CAD build for the part. Positions are in the model's coordinates, mm. Face numbers are marked on the shaded views. A direction names the side the tool comes from. Coordinates: 2 decimals unless noted, no trailing zeros. Loops run counter-clockwise (first coordinate to the right, second up) from the corner with the lowest first, then second, coordinate; pieces in that order, holes last. Notation, with made-up numbers: (-31.5, -5) -> (24.5, -5) arc R16 cw to (24.5, 18) -> close; hole circle Ø8 at (59, 5). An arc over 180 degrees is marked (long way). Write each question's results on one line, items separated by ' | '.
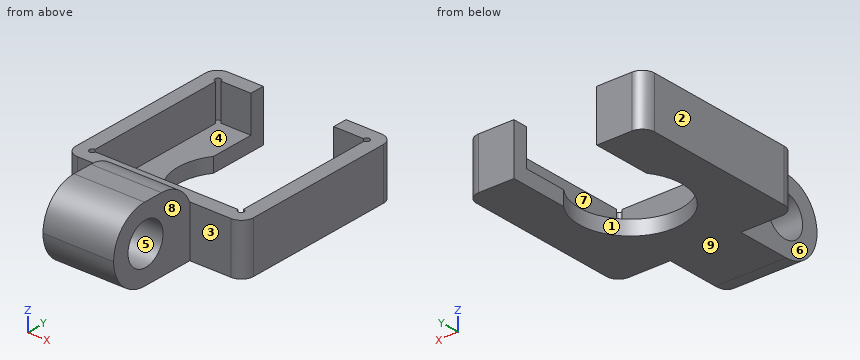
from build123d import *

# Parameters (mm, degrees)
F1_DEPTH    = 1.2
F2_DEPTH    = 4.2
F3_DEPTH    = 6
F6_T1_DEPTH = 20.8
F6_T3_DEPTH = 19.5477270849
F7_D        = 3.4
F7_DEPTH    = 7
F7_TIP      = 1.0214630523
F8_R        = 1


# Not quite as in the source:
# - a fillet or chamfer that OpenCascade refuses, or shapes differently, is made with other operations: its cross-section is extruded or revolved along the edge and cut away or added


with BuildPart() as f1:
    # F0 (on Top) → F1 (new body)
    with BuildSketch(Plane.XY):
        with BuildLine():
            Line((-3.4, 6.1), (-5.85, 6.1))
            ThreePointArc((-5.85, 6.1), (-6.2767766953, 6.2767766953), (-6.1, 5.85))
            Line((-6.1, 5.85), (-6.1, -5.85))
            ThreePointArc((-6.1, -5.85), (-6.2767766953, -6.2767766953), (-5.85, -6.1))
            Line((-5.85, -6.1), (5.85, -6.1))
            ThreePointArc((5.85, -6.1), (6.2767766953, -6.2767766953), (6.1, -5.85))
            Line((6.1, -5.85), (6.1, 5.85))
            ThreePointArc((6.1, 5.85), (6.2767766953, 6.2767766953), (5.85, 6.1))
            Line((5.85, 6.1), (3.4, 6.1))
            Line((3.4, 6.1), (3.4, 2.4657656012))
            ThreePointArc((3.4, 2.4657656012), (0, -4.2), (-3.4, 2.4657656012))
            Line((-3.4, 2.4657656012), (-3.4, 6.1))
        make_face()
    extrude(amount=F1_DEPTH)

    # F0 (on Top) → F2 (join)
    with BuildSketch(Plane.XY):
        with BuildLine():
            ThreePointArc((-6.1, 5.85), (-6.2767766953, 6.2767766953), (-5.85, 6.1))
            Line((-5.85, 6.1), (-3.4, 6.1))
            Line((-3.4, 6.1), (-3.4, 7.3))
            Line((-3.4, 7.3), (-7.3, 7.3))
            Line((-7.3, 7.3), (-7.3, -7.3))
            Line((-7.3, -7.3), (-2.9, -7.3))
            Line((-2.9, -7.3), (2.9, -7.3))
            Line((2.9, -7.3), (7.3, -7.3))
            Line((7.3, -7.3), (7.3, 7.3))
            Line((7.3, 7.3), (3.4, 7.3))
            Line((3.4, 7.3), (3.4, 6.1))
            Line((3.4, 6.1), (5.85, 6.1))
            ThreePointArc((5.85, 6.1), (6.2767766953, 6.2767766953), (6.1, 5.85))
            Line((6.1, 5.85), (6.1, -5.85))
            ThreePointArc((6.1, -5.85), (6.2767766953, -6.2767766953), (5.85, -6.1))
            Line((5.85, -6.1), (-5.85, -6.1))
            ThreePointArc((-5.85, -6.1), (-6.2767766953, -6.2767766953), (-6.1, -5.85))
            Line((-6.1, -5.85), (-6.1, 5.85))
        make_face()
    extrude(amount=F2_DEPTH)

    # F0 (on Top) → F3 (join)
    with BuildSketch(Plane.XY):
        Polygon((2.9, -7.3), (-2.9, -7.3), (-2.9, -14.7), (0, -14.7), (2.9, -14.7), align=None)
    extrude(amount=F3_DEPTH)

    # F6: fillet of radius 3 on 3 edges, made by hand

    # F6_s2 → F6_t1 (cut)
    with BuildSketch(Plane.YZ.offset(-10.4)):
        with BuildLine():
            ThreePointArc((-11.7, 0), (-13.8213203436, 0.8786796564), (-14.7, 3))
            Line((-14.7, 3), (-14.7, 0))
            Line((-14.7, 0), (-11.7, 0))
        make_face()
        with BuildLine():
            ThreePointArc((-11.7, 6), (-13.8213203436, 5.1213203436), (-14.7, 3))
            Line((-14.7, 3), (-14.7, 6))
            Line((-14.7, 6), (-11.7, 6))
        make_face()
    extrude(amount=F6_T1_DEPTH, mode=Mode.SUBTRACT)

    # F6_s4 → F6_t3 (cut)
    with BuildSketch(Plane.YZ.offset(-9.7738635424)):
        with BuildLine():
            ThreePointArc((-7.3, 4.2), (-8.4063777445, 5.5099800796), (-10.049545417, 6))
            Line((-10.049545417, 6), (-7.3, 6))
            Line((-7.3, 6), (-7.3, 4.2))
        make_face()
    extrude(amount=F6_T3_DEPTH, mode=Mode.SUBTRACT)

    # F7
    with Locations(Plane.YZ.offset(3)):
        with Locations((-11.6, 3)):
            Hole(F7_D / 2, depth=F7_DEPTH)
            with Locations((0, 0, -(F7_DEPTH + F7_TIP / 2))):  # 118° drill point
                Cone(0, F7_D / 2, F7_TIP, mode=Mode.SUBTRACT)

    # F8
    f8_edges = [f1.edges().sort_by_distance(p)[0] for p in [
        (-7.3, 7.3, 2.1),
        (-7.3, -7.3, 2.1),
        (7.3, 7.3, 2.1),
        (7.3, -7.3, 2.1),
    ]]
    fillet(f8_edges, radius=F8_R)


solid = f1.part
1) Two-plate mould, pull along X, no slides. Class the marked faces 1, 2, 3 and 4: pulls with the +X half, pulls with the -X half, needs draft (parallel to the pull), parting line crosses it, or undercut.
Outcome:
face 1: undercut | face 2: pulls with the -X half | face 3: needs draft | face 4: undercut
2) Pin check, flat tips, straight feed: pin 1 (4 mm diameter, centred on x = -1, y = -7.5, fed in from +Z); pin 2 (7.5 mm diameter, centred on x = 3.5, y = 1.5, fed in from +Z); pin 3 (6.5 mm diameter, centred on x = 1, y = -0.5, fed in from +Z). Stop position of each tip, or through.
Outcome:
pin 1: stops at z = 5.95 | pin 2: stops at z = 4.2 | pin 3: stops at z = 1.2
3) Slice it at A-A (y = 5). Write the cut outline in (x, z), then the cut area to 3 significant figures.
Outcome:
outline: (-7.3, 0) -> (-3.4, 0) -> (-3.4, 1.2) -> (-6.1, 1.2) -> (-6.1, 4.2) -> (-7.3, 4.2) -> close; (3.4, 0) -> (7.3, 0) -> (7.3, 4.2) -> (6.1, 4.2) -> (6.1, 1.2) -> (3.4, 1.2) -> close | area: 16.6 mm^2
4) Slice it at D-D (x = -5.25). Write the cut outline in (y, z).
Outcome:
outline: (-7.3, 0) -> (7.3, 0) -> (7.3, 4.2) -> (6.1, 4.2) -> (6.1, 1.2) -> (-6.1, 1.2) -> (-6.1, 4.2) -> (-7.3, 4.2) -> close
5) Slice it at C-C (z = 2.5). Write the cut outline in (x, y).
Outcome:
outline: (-7.3, -6.3) arc R1 ccw to (-6.3, -7.3) -> (-2.9, -7.3) -> (-2.9, -9.98) -> (2.9, -9.98) -> (2.9, -7.3) -> (6.3, -7.3) arc R1 ccw to (7.3, -6.3) -> (7.3, 6.3) arc R1 ccw to (6.3, 7.3) -> (3.4, 7.3) -> (3.4, 6.1) -> (5.85, 6.1) arc R0.25 cw (long way) to (6.1, 5.85) -> (6.1, -5.85) arc R0.25 cw (long way) to (5.85, -6.1) -> (-5.85, -6.1) arc R0.25 cw (long way) to (-6.1, -5.85) -> (-6.1, 5.85) arc R0.25 cw (long way) to (-5.85, 6.1) -> (-3.4, 6.1) -> (-3.4, 7.3) -> (-6.3, 7.3) arc R1 ccw to (-7.3, 6.3) -> close; (-2.9, -14.66) -> (2.9, -14.66) -> (2.9, -13.22) -> (-2.9, -13.22) -> close
6) Slice it at B-B (x = 0). Write the cut outline in (y, z).
Outcome:
outline: (-11.7, 0) -> (-4.2, 0) -> (-4.2, 1.2) -> (-6.1, 1.2) -> (-6.1, 4.2) -> (-7.3, 4.2) arc R3 ccw to (-10.05, 6) -> (-11.7, 6) arc R3 ccw to start; hole circle Ø3.4 at (-11.6, 3)
7) Which spindle directions (+Z, -Z, +X, -X, +Y, -Y) get a long thin tool onto all of the face, cutting with end or side? Do the marked faces 5, 6, 7, 8 and 9. Say none if no direction does.
Outcome:
face 5: +X, -X | face 6: +Z, -Z, -X, -Y | face 7: +Z | face 8: +Z, -Z, +X, -Y | face 9: -Z, +X, -X, +Y, -Y
8) Drill centre lines: L1, parallel to Y at x = -4, z = 1.25; L2, parallel to Z at x = -0.75, y = -11.5; L3, parallel to X at y = 0, z = 0.45. Where is each one in solid material? Low to high. Write a range as from..to.
Outcome:
L1: y = -7.3..-6.1, 6.1..7.3 | L2: z = 0..1.3, 4.7..6 | L3: x = -7.3..-4.2, 4.2..7.3
